Can you work these out from the model? Positions are in its coordinate system, mm. Coordinates: 2 decimals unless noted, no trailing zeros. Loops run counter-clockwise (first coordinate to the right, second up) from the corner with the lowest first, then second, coordinate; pieces in that order, holes last. Notation, with made-up numbers: (43, -8) -> (86, -8) arc R23 cw to (86, 27) -> close; hole circle Ø6 at (77, 53). An arc over 180 degrees is marked (long way). Put each result on its own line as item: value. Start each with the question number.
Item 1: If we section it at C-C on z = 9.25: Please give me the cut outline in (x, y).
Item 2: We'd pull the mould along Z, two halves only. Please class faces 1 (the flat face through (0, -134, 5)), 2 (the cylindrical face through (1.878, -13.75, 12.875)): pulls with the +Z half, pulls with the -Z half, needs draft (parallel to the pull), parting line crosses it, or undercut.
Item 3: If we section it at B-B on y = -227: Please give me the cut outline in (x, z).
Item 4: Will these pins go through, and if not, where does the flat tip stop? P1, Ø4, axis at y = -14.92, z = 15.13, coming from the +X side; P2, Ø1.9, axis at x = 1.5, z = 8.5, coming from the +Y side.
Item 5: If we section it at A-A on x = 3.2: Please give me the cut outline in (y, z), plus the area to 3 significant figures.
Item 6: Please list where these lines run through material, in increasing order: L1, parallel to Y at x = 0.8, z = 15.25; L2, parallel to Z at x = 3.1, y = -84; L3, parallel to Y at x = 1, z = 12.25. Write a range as from..to.
```python
from build123d import *

# Parameters (mm, degrees)
F0_R          = 2.54
F1_DEPTH      = 3.81
F1_FACE_W     = 3.81
F1_FACE_H     = 7.62
F2_DEPTH      = 7.62
F3_W          = 3.81
F3_H          = 2.54
F4_DEPTH      = 254
F4_DEPTH_BACK = 25.4


with BuildPart() as f1:
    # F0 (on Right) → F1 (new body)
    with BuildSketch(Plane.YZ):
        with BuildLine():
            ThreePointArc((-11.112122, 15.191537), (-14.922122, 18.938949), (-18.732122, 15.191537))
            Line((-18.732122, 15.191537), (-18.732122, 11.381537))
            Line((-18.732122, 11.381537), (-11.112122, 11.381537))
            Line((-11.112122, 11.381537), (-11.112122, 15.191537))
        make_face()
        with Locations((-14.922122, 15.128426)):
            Circle(F0_R, mode=Mode.SUBTRACT)
    extrude(amount=F1_DEPTH)

    # F1_face (on face) → F2 (join)
    with BuildSketch(Plane(origin=(1.905, -14.922122, 11.381537), x_dir=(1, 0, 0), z_dir=(0, 0, -1))):
        Rectangle(F1_FACE_W, F1_FACE_H)
    extrude(amount=F2_DEPTH)

    # F3 (on face) → F4 (join, two sides)
    with BuildSketch(Plane.XZ.offset(18.732122)) as f4_sk:
        with Locations((1.905, 5.031537)):
            Rectangle(F3_W, F3_H)
    extrude(amount=F4_DEPTH)
    extrude(f4_sk.sketch, amount=-F4_DEPTH_BACK)


solid = f1.part
```
Solutions:
1. outline: (0, -18.73) -> (3.81, -18.73) -> (3.81, -11.11) -> (0, -11.11) -> close
2. face 1: needs draft
2. face 2: undercut
3. outline: (0, 3.76) -> (3.81, 3.76) -> (3.81, 6.3) -> (0, 6.3) -> close
4. P1: through
4. P2: y = -11.11
5. outline: (-272.73, 3.76) -> (6.67, 3.76) -> (6.67, 6.3) -> (-11.11, 6.3) -> (-11.11, 15.19) arc R3.81 ccw to (-18.73, 15.19) -> (-18.73, 6.3) -> (-272.73, 6.3) -> close; hole circle Ø5.08 at (-14.92, 15.13)
5. area: 779 mm^2
6. L1: -18.73..-17.46, -12.39..-11.11
6. L2: 3.76..6.3
6. L3: -18.73..-11.11
